Source: CAD feature listing. Evaluate the final solid. Frame: model axes, mm. Face numbers are marked on the shaded views. A direction names the side the tool comes from. Give positions to 0.01 mm unless a question says otherwise; leave off trailing zeros. Order: outer loops, then holes, each group sorted by start corner. A loop starts at its lowest first (then second) coordinate and runs counter-clockwise, first axis right, second up.
from build123d import *

# Parameters (mm, degrees)
ESQUISSE1_W             = 20
ESQUISSE1_H             = 20
BOSS_EXTRU_1_DEPTH      = 5
ESQUISSE2_W             = 15
ESQUISSE2_H             = 15
BOSS_EXTRU_2_DEPTH      = 35
ESQUISSE3_R             = 0.75
ENL_V_MAT_EXTRU_1_DEPTH = 5
ESQUISSE5_W             = 15
ESQUISSE5_H             = 5
BOSS_EXTRU_3_DEPTH      = 40
ENL_V_MAT_EXTRU_2_DEPTH = 5
CONG_1_R                = 1


with BuildPart() as part:
    # Esquisse1 → Boss.-Extru.1 (new body)
    with BuildSketch(Plane(origin=(0, 0, 0), x_dir=(1, 0, 0), z_dir=(0, 1, 0))):
        Rectangle(ESQUISSE1_W, ESQUISSE1_H)
    extrude(amount=BOSS_EXTRU_1_DEPTH)

    # Esquisse2 → Boss.-Extru.2 (add)
    with BuildSketch(Plane(origin=(0, 0, 0), x_dir=(-1, 0, 0), z_dir=(0, -1, 0))):
        Rectangle(ESQUISSE2_W, ESQUISSE2_H)
    extrude(amount=-BOSS_EXTRU_2_DEPTH)

    # Esquisse3 → Enlèv. mat.-Extru.1 (cut)
    with BuildSketch(Plane(origin=(0, 5, 0), x_dir=(1, 0, 0), z_dir=(0, 1, 0))):
        with Locations((-8.75, 0)):
            Circle(ESQUISSE3_R)
        with Locations((0, 8.75)):
            Circle(ESQUISSE3_R)
        with Locations((8.75, 0)):
            Circle(ESQUISSE3_R)
        with Locations((0, -8.75)):
            Circle(ESQUISSE3_R)
    extrude(amount=-ENL_V_MAT_EXTRU_1_DEPTH, mode=Mode.SUBTRACT)

    # Esquisse5 → Boss.-Extru.3 (add)
    with BuildSketch(Plane(origin=(7.5, 0, 0), x_dir=(0, 0, -1), z_dir=(1, 0, 0))):
        with Locations((0, 32.5)):
            Rectangle(ESQUISSE5_W, ESQUISSE5_H)
    extrude(amount=BOSS_EXTRU_3_DEPTH)

    # Esquisse6 → Enlèv. mat.-Extru.2 (cut)
    with BuildSketch(Plane(origin=(0, 35, 0), x_dir=(1, 0, 0), z_dir=(0, 1, 0))):
        Polygon((10, 7.5), (36.497560734, 0.4), (47.5, 0.4), (47.5, 7.5), align=None)
        Polygon((36.497560734, -0.4), (47.5, -0.4), (47.5, -7.5), (10, -7.5), align=None)
    extrude(amount=-ENL_V_MAT_EXTRU_2_DEPTH, mode=Mode.SUBTRACT)

    # Congé1
    cong_1_edges = [part.edges().sort_by_distance(p)[0] for p in [
        (7.5, 30, 0),
        (36.497560734, 32.5, -0.4),
        (36.497560734, 32.5, 0.4),
    ]]
    fillet(cong_1_edges, radius=CONG_1_R)


solid = part.part
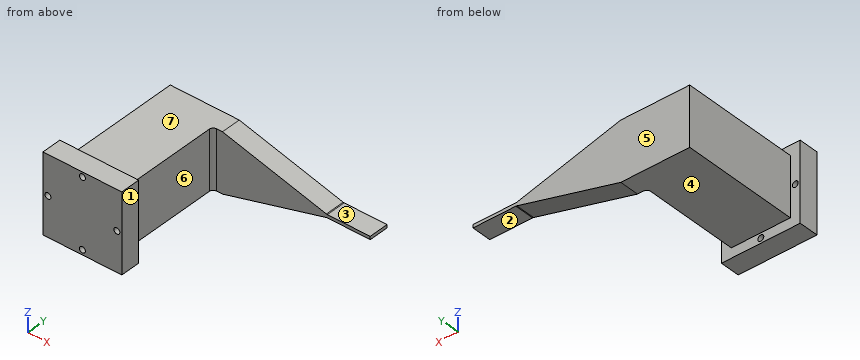
1) Pull-direction query (Y, two-part tool) for the marked faces 5, 6 and 7; classes: +Y half, -Y half, draft (parallel to the pull), parting line (faces both ways), or undercut.
Checks:
face 5: +Y half
face 6: undercut
face 7: draft
2) Section query A-A on z = -8.75. Output: boundary loops of the cut face in (x, y).
Checks:
outline: (-10, 0) - (-0.75, 0) - (-0.75, 5) - (-10, 5) - close; (0.75, 0) - (10, 0) - (10, 5) - (0.75, 5) - close
3) Reachability of the marked faces 1, 2, 3 and 4 from +Z, -Z, +X, -X, +Y, -Y: full face, straight path, thin tool, end or side. Return the list, or none.
Checks:
face 1: +Z, -Z, +X, -Y
face 2: -Z, +X, +Y, -Y
face 3: +Z, +X, +Y, -Y
face 4: -Z, +X, -X, +Y
4) Section query D-D on y = 28. Output: boundary loops of the cut face in (x, z).
Checks:
outline: (-7.5, -7.5) - (7.5, -7.5) - (7.5, 7.5) - (-7.5, 7.5) - close
5) First-contact query: pin 1 Ø1.5 at (x, z) = (14, 6.5) entering from +Y; pin 2 Ø4.5 at (x, z) = (19, -3.5) entering from -Y; pin 3 Ø4 at (y, z) = (12.5, 0) entering from +X; pin 4 Ø19 at (x, y) = (1.5, 16.5) entering from +Z. Flat tips, straight axial feed; report the tip coordinate or a pass-through.
Checks:
pin 1: stops at y = 35
pin 2: stops at y = 30
pin 3: stops at x = 7.5
pin 4: stops at z = 7.5
6) Section query C-C on x = 2. Output: boundary loops of the cut face in (y, z).
Checks:
outline: (0, -10) - (5, -10) - (5, -7.5) - (35, -7.5) - (35, 7.5) - (5, 7.5) - (5, 10) - (0, 10) - close
7) Section query B-B on x = -8.75. Output: boundary loops of the cut face in (y, z).
Checks:
outline: (0, -10) - (5, -10) - (5, -0.75) - (0, -0.75) - close; (0, 0.75) - (5, 0.75) - (5, 10) - (0, 10) - close
8) Ray query, L1, parallel to X at y = 3.8, z = 0; L2, parallel to X at y = 4, z = 8.75. Return the intervals inside material, ascending.
Checks:
L1: x = -10 to -9.5, -8 to 8, 9.5 to 10
L2: x = -10 to -0.75, 0.75 to 10
